Work out the finished part from the listing and answer in its coordinate system (mm). Face numbers are marked on the shaded views. Give positions to 0.01 mm unless a question says otherwise; leave off trailing zeros. Order: outer loops, then holes, each group sorted by start corner. A loop starts at its lowest first (then second) coordinate and runs counter-clockwise, first axis right, second up. Notation, with made-up numbers: (20.25, 18.5) - (30.25, 18.5) arc R21 cw to (30.25, 30.5) - close; hole circle Ø3 at (23, 5). An arc over 180 degrees is marked (long way). Put each result on its own line as item: value.
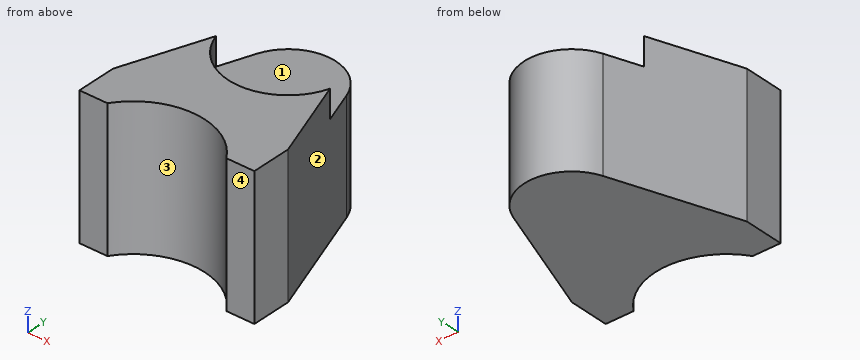
```python
from build123d import *

# Parameters (mm, degrees)
BOSS_EXTRUDE1_DEPTH = 17.5
SKETCH2_R           = 15
CUT_EXTRUDE1_DEPTH  = 7


with BuildPart() as part:
    # Sketch1 → Boss-Extrude1 (new, symmetric)
    with BuildSketch(Plane.XY):
        with BuildLine():
            Line((14.966629547, 0), (22, 0))
            Line((22, 0), (22, 10))
            Line((22, 10), (11.304244422, 40.026668357))
            ThreePointArc((11.304244422, 40.026668357), (0, 48), (-11.304244422, 40.026668357))
            Line((-11.304244422, 40.026668357), (-22, 10))
            Line((-22, 10), (-22, 0))
            Line((-22, 0), (-14.966629547, 0))
            ThreePointArc((-14.966629547, 0), (0, 8), (14.966629547, 0))
        make_face()
    extrude(amount=BOSS_EXTRUDE1_DEPTH, both=True)

    # Sketch2 → Cut-Extrude1 (cut)
    with BuildSketch(Plane.XY.offset(17.5)):
        with Locations((0, 36)):
            Circle(SKETCH2_R)
    extrude(amount=-CUT_EXTRUDE1_DEPTH, mode=Mode.SUBTRACT)


solid = part.part
```
(1) Straight lines are drawn through the part: line 1 (Z direction, x = 6.5, y = 44); line 2 (X direction, y = 5, z = -14); line 3 (X direction, y = 13, z = 1.5). For each, find the intervals that lie inside material, in ascending order.
Geometry check:
line 1: z = -17.5 to 10.5
line 2: x = -22 to -9.95, 9.95 to 22
line 3: x = -20.93 to 20.93
(2) Section D-D, the plane x = -13 is taken. Write down the section's boundary in (y, z), then the cut area to 3 significant figures.
Geometry check:
outline: (2.45, -17.5) - (35.27, -17.5) - (35.27, 10.5) - (28.52, 10.5) - (28.52, 17.5) - (2.45, 17.5) - close
area: 1,100 mm²
(3) Section B-B, the plane y = 27 is taken. Write down the section's boundary in (x, z).
Geometry check:
outline: (-15.94, -17.5) - (15.94, -17.5) - (15.94, 17.5) - (12, 17.5) - (12, 10.5) - (-12, 10.5) - (-12, 17.5) - (-15.94, 17.5) - close
(4) Given pin 1 (3 mm diameter, centred on x = -4.5, y = 28.5, fed in from +Z); pin 2 (2 mm diameter, centred on y = 38.5, z = -12.5, fed in from +X); pin 3 (5 mm diameter, centred on x = -13, z = -12.5, fed in from +Y), each flat-ended and moving along its own axis, determine where each tip first touches the part or whether it passes through.
Geometry check:
pin 1: stops at z = 10.5
pin 2: stops at x = 12.2
pin 3: stops at y = 41.81
(5) Section C-C, the plane x = -2 is taken. Write down the section's boundary in (y, z), then the cut area to 3 significant figures.
Geometry check:
outline: (7.89, -17.5) - (47.83, -17.5) - (47.83, 10.5) - (21.13, 10.5) - (21.13, 17.5) - (7.89, 17.5) - close
area: 1,210 mm²
(6) Determine the mould class of the marked faces 1, 2, 3 and 4 for opening direction X: pulls with the +X half, pulls with the -X half, needs draft (parallel to the pull), parting line crosses it, or undercut.
Geometry check:
face 1: undercut
face 2: pulls with the +X half
face 3: undercut
face 4: needs draft
(7) Section A-A, the plane z = -5 is taken. Write down the section's boundary in (x, y), then the cut area to 3 significant figures.
Geometry check:
outline: (-22, 0) - (-14.97, 0) arc R18 cw to (14.97, 0) - (22, 0) - (22, 10) - (11.3, 40.03) arc R12 ccw to (-11.3, 40.03) - (-22, 10) - close
area: 1,400 mm²
